Could you check a few things on this model? Use its own coordinates, in mm. A direction names the side the tool comes from. Coordinates: 2 decimals unless noted, no trailing zeros.
Item 1: Thinking about a two-plate mould opening in Y: for faces 4 (the cylindrical face through (-6.806, -3.608, -4.436)), 5 (the cylindrical face through (-0.765, -1.225, 2.031)), which applies, +Y half, -Y half, draft (parallel to the pull), parting line (faces both ways), or undercut?
Item 2: I want a section at A-A on z = 2. State how many separate pieces and enclosed holes the cut face has, then the cut area to 3 significant figures.
Item 3: If I drill on probe 1 along Z at (x, y) = (8, -2.25); probe 2 along Y at (x, z) = (-5, -3.5); probe 3 along X at (y, z) = (-1, 3), over which ranges is the centre line in solid material (lowest first)?
Item 4: For P1, Ø1, axis at y = -3, z = 2, coming from the -X side; P2, Ø3, axis at y = -1.5, z = 4, coming from the -X side; P3, Ø0.6, axis at x = -5.5, y = 1.5, coming from the +Z side, each with a flat end and sliding along its axis, tell me the tip position at first contact or that it passes through.
Item 5: Which directions (+Z, -Z, +X, -X, +Y, -Y) give clear straight access to the entire face, cutting with the end or side of a thin tool? Please do faces 1 (the cylindrical face through (-0.152, 0.737, -5.696)), 2 (the flat face through (3, 1, -2)), 3 (the flat face through (0, -3.535, 3)).
from build123d import *

# Parameters (mm, degrees)
ARRAY008_X_COUNT = 5
ARRAY008_X_PITCH = 2.77
ARRAY007_X_COUNT = 4
ARRAY007_X_PITCH = 2.77
ARRAY007_Y_COUNT = 2
ARRAY007_Y_PITCH = 100
PAD004_DEPTH     = 3.45
PAD005_DEPTH     = 2
FILLET007_R      = 0.7
PAD008_DEPTH     = 6.55
SKETCH016_R      = 0.7
PAD006_DEPTH     = 0.5
ARRAY_X_COUNT    = 5
ARRAY_X_PITCH    = 2.77
SKETCH017_R      = 0.7
PAD007_DEPTH     = 0.5
ARRAY001_X_COUNT = 4
ARRAY001_X_PITCH = 2.77


with BuildPart() as array008:
    # Sketch025 → Revolution008 (revolve)
    with BuildSketch(Plane.XZ):
        with BuildLine():
            Line((0, 6.65), (0, -10.75))
            ThreePointArc((0, -10.75), (0.212132, -10.662132), (0.3, -10.45))
            Line((0.3, -10.45), (0.3, -2))
            Line((0.3, -2), (0.65, -2))
            Line((0.65, -2), (0.65, 5.95))
            Line((0.65, 5.95), (1.35, 6.65))
            Line((1.35, 6.65), (0, 6.65))
        make_face()
    revolve(axis=Axis((0, 0, 0), (0, 0, 1)))


with BuildPart() as array008_1:
    # Body015 placement: moved
    add(array008.part.moved(Location((-5.54, 1.42, 0))))

    # Array008 X: Array008 ×5


with BuildPart() as array008_2:
    add(array008_1.part)
    with Locations(*[(i * ARRAY008_X_PITCH, 0, 0) for i in range(1, ARRAY008_X_COUNT)]):
        add(array008_1.part)


with BuildPart() as fusion003:
    # Sketch024 → Revolution007 (revolve)
    with BuildSketch(Plane.XZ):
        with BuildLine():
            Line((0, 6.65), (0, -10.75))
            ThreePointArc((0, -10.75), (0.212132, -10.662132), (0.3, -10.45))
            Line((0.3, -10.45), (0.3, -2))
            Line((0.3, -2), (0.65, -2))
            Line((0.65, -2), (0.65, 5.95))
            Line((0.65, 5.95), (1.35, 6.65))
            Line((1.35, 6.65), (0, 6.65))
        make_face()
    revolve(axis=Axis((0, 0, 0), (0, 0, 1)))


with BuildPart() as fusion003_1:
    # Body014 placement: moved
    add(fusion003.part.moved(Location((-4.155, -1.42, 0))))

    # Array007 X: Fusion003 ×4


with BuildPart() as fusion003_2:
    add(fusion003_1.part)
    with Locations(*[(i * ARRAY007_X_PITCH, 0, 0) for i in range(1, ARRAY007_X_COUNT)]):
        add(fusion003_1.part)

    # Array007 Y: Fusion003 ×2


with BuildPart() as fusion003_3:
    add(fusion003_2.part)
    with Locations(*[(0, i * ARRAY007_Y_PITCH, 0) for i in range(1, ARRAY007_Y_COUNT)]):
        add(fusion003_2.part)

    # Fusion003: union Array008
    add(array008_2.part)


with BuildPart() as body006:
    # Sketch014 → Pad004 (new body)
    with BuildSketch(Plane.XY):
        with BuildLine():
            Line((-5.72, 5), (5.72, 5))
            ThreePointArc((9.068211, 1.008831), (8.324801, 3.78518), (5.72, 5))
            Line((9.068211, 1.008831), (8.503211, -2.191169))
            ThreePointArc((5.155, -5), (7.34018, -4.204801), (8.503211, -2.191169))
            Line((5.155, -5), (-5.155, -5))
            ThreePointArc((-8.503211, -2.191169), (-7.34018, -4.204801), (-5.155, -5))
            Line((-8.503211, -2.191169), (-9.068211, 1.008831))
            ThreePointArc((-5.72, 5), (-8.324801, 3.78518), (-9.068211, 1.008831))
        make_face()
    extrude(amount=-PAD004_DEPTH)

    # Sketch015 (on Face10 of Pad004) → Pad005 (join)
    with BuildSketch(Plane(origin=(0, 0, -3.45), x_dir=(1, 0, 0), z_dir=(0, 0, -1))):
        with BuildLine():
            Line((-5.155, 4.2), (5.155, 4.2))
            ThreePointArc((7.715397, 2.05207), (6.82602, 3.591906), (5.155, 4.2))
            Line((7.715397, 2.05207), (8.280397, -1.14793))
            ThreePointArc((5.72, -4.2), (7.711906, -3.27102), (8.280397, -1.14793))
            Line((5.72, -4.2), (-5.72, -4.2))
            ThreePointArc((-8.280397, -1.14793), (-7.711906, -3.27102), (-5.72, -4.2))
            Line((-8.280397, -1.14793), (-7.715397, 2.05207))
            ThreePointArc((-5.155, 4.2), (-6.82602, 3.591906), (-7.715397, 2.05207))
        make_face()
    extrude(amount=PAD005_DEPTH)

    # Fillet007
    fillet007_edges = [body006.edges().sort_by_distance(p)[0] for p in [
        (-8.785711, -0.591169, -3.45),
    ]]
    fillet(fillet007_edges, radius=FILLET007_R)

    # Sketch022 (on Face4 of Fillet007) → Pad008 (join)
    with BuildSketch(Plane.XY):
        with BuildLine():
            Line((-5.475, 3.535), (5.475, 3.535))
            ThreePointArc((7.587437, 1.017664), (7.11812, 2.768834), (5.475, 3.535))
            Line((7.587437, 1.017664), (7.097437, -1.762336))
            ThreePointArc((4.985, -3.535), (6.363834, -3.03312), (7.097437, -1.762336))
            Line((4.985, -3.535), (-4.985, -3.535))
            ThreePointArc((-7.097437, -1.762336), (-6.363834, -3.03312), (-4.985, -3.535))
            Line((-7.097437, -1.762336), (-7.587437, 1.017664))
            ThreePointArc((-5.475, 3.535), (-7.11812, 2.768834), (-7.587437, 1.017664))
        make_face()
    extrude(amount=PAD008_DEPTH)


with BuildPart() as array:
    # Sketch016 → Pad006 (new body)
    with BuildSketch(Plane.XY):
        Circle(SKETCH016_R)
    extrude(amount=-PAD006_DEPTH)


with BuildPart() as array_1:
    # Body007 placement: moved
    add(array.part.moved(Location((-5.54, 1.42, -5.45))))

    # Array X: Array ×5


with BuildPart() as array_2:
    add(array_1.part)
    with Locations(*[(i * ARRAY_X_PITCH, 0, 0) for i in range(1, ARRAY_X_COUNT)]):
        add(array_1.part)


with BuildPart() as cut:
    # Sketch017 → Pad007 (new body)
    with BuildSketch(Plane.XY):
        Circle(SKETCH017_R)
    extrude(amount=-PAD007_DEPTH)


with BuildPart() as cut_1:
    # Body008 placement: moved
    add(cut.part.moved(Location((-4.155, -1.42, -5.45))))

    # Array001 X: Cut ×4


with BuildPart() as cut_2:
    add(cut_1.part)
    with Locations(*[(i * ARRAY001_X_PITCH, 0, 0) for i in range(1, ARRAY001_X_COUNT)]):
        add(cut_1.part)

    # Fusion: union Array
    add(array_2.part)

    # Fusion002: union Body006
    add(body006.part)

    # Cut: cut Fusion003
    add(fusion003_3.part, mode=Mode.SUBTRACT)


solid = cut_2.part
Response values:
1. face 4: -Y half
1. face 5: undercut
2. separate pieces: 1
2. enclosed holes: 9
2. area: 88.6 mm2
3. probe 1: z = -3.42 to 0
3. probe 2: y = -4.2 to 4.2
3. probe 3: x = -7.23 to -4.65, -3.66 to -1.88, -0.89 to 0.89, 1.88 to 3.66, 4.65 to 7.23
4. P1: stops at x = -6.82
4. P2: stops at x = -7.41
4. P3: stops at z = -2
5. face 1: -Z
5. face 2: +Z
5. face 3: +Z, +X, -X, -Y
